Input: dimensioned drawing with shaded views. Units: mm. Origin: part minimum x, y, z. Coordinates: 2 decimals unless noted, no trailing zeros. Order: outer loops, then holes, each group sorted by start corner. A loop starts at its lowest first (then second) coordinate and runs counter-clockwise, first axis right, second up. Notation, with made-up numbers: (1, 61.5) - (20, 61.5) arc R30 cw to (20, 85.5) - close; hole circle Ø7 at (-39.5, -25.5). An arc over 180 degrees is marked (long way). Use one line per item in the form item = value. Start each with the question number.
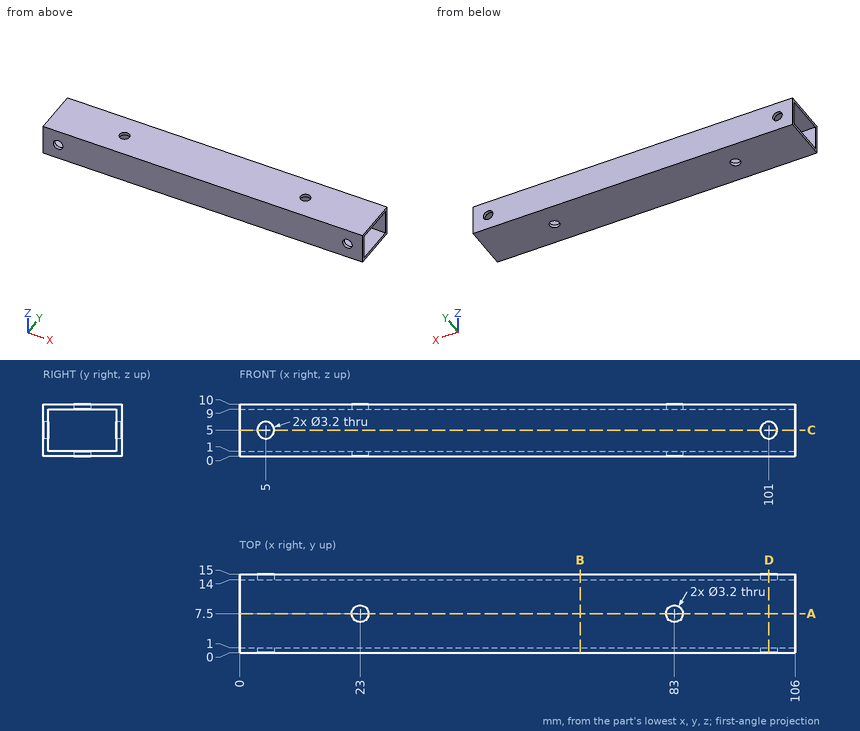
(1) Material intervals for L1, parallel to X at y = 7.5, z = 0.75; L2, parallel to Z at x = 40, y = 6.5; L3, parallel to Y at x = 101, z = 7.25, sorted ascending. Write a range as from..to.
(2) Cut plane B-B on x = 65. Return the cut outline in (y, z).
(3) Cut plane C-C on z = 5. Return the cut outline in (x, y).
(4) Cut plane D-D on x = 101. Return the cut outline in (y, z), plus the area to 3 significant figures.
(5) Cut plane A-A on y = 7.5. Return the cut outline in (x, z).
Check sheet entries:
q1.L1 = 0..21.4, 24.6..81.4, 84.6..106
q1.L2 = 0..1, 9..10
q1.L3 = 0..1, 14..15
q2.outline = (0, 0) - (15, 0) - (15, 10) - (0, 10) - close; hole (1, 1) - (14, 1) - (14, 9) - (1, 9) - close
q3.outline = (0, 0) - (3.4, 0) - (3.4, 1) - (0, 1) - close; (0, 14) - (3.4, 14) - (3.4, 15) - (0, 15) - close; (6.6, 0) - (99.4, 0) - (99.4, 1) - (6.6, 1) - close; (6.6, 14) - (99.4, 14) - (99.4, 15) - (6.6, 15) - close; (102.6, 0) - (106, 0) - (106, 1) - (102.6, 1) - close; (102.6, 14) - (106, 14) - (106, 15) - (102.6, 15) - close
q4.outline = (0, 0) - (15, 0) - (15, 3.4) - (14, 3.4) - (14, 1) - (1, 1) - (1, 3.4) - (0, 3.4) - close; (0, 6.6) - (1, 6.6) - (1, 9) - (14, 9) - (14, 6.6) - (15, 6.6) - (15, 10) - (0, 10) - close
q4.area = 39.6 mm^2
q5.outline = (0, 0) - (21.4, 0) - (21.4, 1) - (0, 1) - close; (0, 9) - (21.4, 9) - (21.4, 10) - (0, 10) - close; (24.6, 0) - (81.4, 0) - (81.4, 1) - (24.6, 1) - close; (24.6, 9) - (81.4, 9) - (81.4, 10) - (24.6, 10) - close; (84.6, 0) - (106, 0) - (106, 1) - (84.6, 1) - close; (84.6, 9) - (106, 9) - (106, 10) - (84.6, 10) - close
